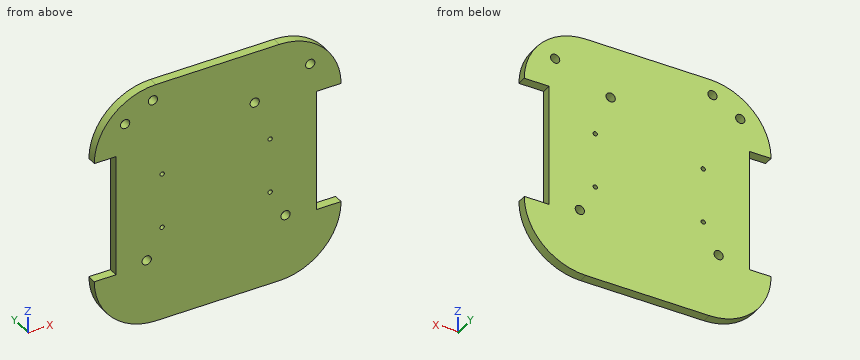
from build123d import *

# Parameters (mm, degrees)
SKETCH3_W           = 80
SKETCH3_H           = 80
BOSS_EXTRUDE1_DEPTH = 3
SKETCH4_W           = 7
SKETCH4_H           = 40
SKETCH4_W_2         = 8
CUT_EXTRUDE1_DEPTH  = 3
FILLET3_R           = 20
FILLET4_R           = 20
FILLET5_R           = 20
FILLET6_R           = 20
SKETCH6_R           = 1.5
CUT_EXTRUDE2_DEPTH  = 3
SKETCH9_R           = 1.5
CUT_EXTRUDE3_DEPTH  = 3
SKETCH10_R          = 1.5
CUT_EXTRUDE4_DEPTH  = 3
SKETCH11_R          = 0.7
CUT_EXTRUDE5_DEPTH  = 3


with BuildPart() as part:
    # Sketch3 → Boss-Extrude1 (new body)
    with BuildSketch(Plane(origin=(0, 0, 0), x_dir=(1, 0, 0), z_dir=(0, 1, 0))):
        with Locations((40, 40)):
            Rectangle(SKETCH3_W, SKETCH3_H)
    extrude(amount=BOSS_EXTRUDE1_DEPTH)

    # Sketch4 → Cut-Extrude1 (cut)
    with BuildSketch(Plane(origin=(0, 3, 0), x_dir=(1, 0, 0), z_dir=(0, 1, 0))):
        with Locations((3.5, 40)):
            Rectangle(SKETCH4_W, SKETCH4_H)
        with Locations((76, 40)):
            Rectangle(SKETCH4_W_2, SKETCH4_H)
    extrude(amount=-CUT_EXTRUDE1_DEPTH, mode=Mode.SUBTRACT)

    # Fillet3
    fillet3_edges = [part.edges().sort_by_distance(p)[0] for p in [
        (0, 1.5, -80),
    ]]
    fillet(fillet3_edges, radius=FILLET3_R - 0.0001)  # a hair under: the kernel refuses the full size

    # Fillet4
    fillet4_edges = [part.edges().sort_by_distance(p)[0] for p in [
        (80, 1.5, -80),
    ]]
    fillet(fillet4_edges, radius=FILLET4_R - 0.0001)  # a hair under: the kernel refuses the full size

    # Fillet5
    fillet5_edges = [part.edges().sort_by_distance(p)[0] for p in [
        (80, 1.5, 0),
    ]]
    fillet(fillet5_edges, radius=FILLET5_R - 0.0001)  # a hair under: the kernel refuses the full size

    # Fillet6
    fillet6_edges = [part.edges().sort_by_distance(p)[0] for p in [
        (0, 1.5, 0),
    ]]
    fillet(fillet6_edges, radius=FILLET6_R - 0.0001)  # a hair under: the kernel refuses the full size

    # Sketch6 → Cut-Extrude2 (cut)
    with BuildSketch(Plane(origin=(0, 3, 0), x_dir=(1, 0, 0), z_dir=(0, 1, 0))):
        with Locations(Location((17, 58.5, 0), (0, 0, 270))):
            Circle(SKETCH6_R)
        with Locations(Location((62, 58.5, 0), (0, 0, 270))):
            Circle(SKETCH6_R)
    extrude(amount=-CUT_EXTRUDE2_DEPTH, mode=Mode.SUBTRACT)

    # Sketch9 → Cut-Extrude3 (cut)
    with BuildSketch(Plane(origin=(0, 3, 0), x_dir=(1, 0, 0), z_dir=(0, 1, 0))):
        with Locations(Location((70, 10, 0), (0, 0, 270))):
            Circle(SKETCH9_R)
        with Locations(Location((10, 10, 0), (0, 0, 270))):
            Circle(SKETCH9_R)
    extrude(amount=-CUT_EXTRUDE3_DEPTH, mode=Mode.SUBTRACT)

    # Sketch10 → Cut-Extrude4 (cut)
    with BuildSketch(Plane(origin=(0, 3, 0), x_dir=(1, 0, 0), z_dir=(0, 1, 0))):
        with Locations(Location((19, 5, 0), (0, 0, 270))):
            Circle(SKETCH10_R)
        with Locations(Location((52, 17, 0), (0, 0, 270))):
            Circle(SKETCH10_R)
    extrude(amount=-CUT_EXTRUDE4_DEPTH, mode=Mode.SUBTRACT)

    # Sketch11 → Cut-Extrude5 (cut)
    with BuildSketch(Plane(origin=(0, 3, 0), x_dir=(1, 0, 0), z_dir=(0, 1, 0))):
        with Locations(Location((22, 49, 0), (0, 0, 270))):
            Circle(SKETCH11_R)
        with Locations(Location((22, 31, 0), (0, 0, 270))):
            Circle(SKETCH11_R)
        with Locations(Location((57, 49, 0), (0, 0, 270))):
            Circle(SKETCH11_R)
        with Locations(Location((57, 31, 0), (0, 0, 270))):
            Circle(SKETCH11_R)
    extrude(amount=-CUT_EXTRUDE5_DEPTH, mode=Mode.SUBTRACT)


solid = part.part
Design review of the part built by this model. Coordinates are the model's own, in mm. Coordinates: 2 decimals unless noted, no trailing zeros. Loops run counter-clockwise (first coordinate to the right, second up) from the corner with the lowest first, then second, coordinate; pieces in that order, holes last.
Item 1: Add section A-A (y = 1.6). Give the number of separate pieces and of enclosed holes in the cut face, and give its area (3 significant figures).
Completed:
separate pieces: 1
enclosed holes: 10
area: 5,410 mm2
Item 2: Add section B-B (x = 52). Write out the cut boundary in (y, z).
Completed:
outline: (0, -80) - (3, -80) - (3, -18.5) - (0, -18.5) - close; (0, -15.5) - (3, -15.5) - (3, 0) - (0, 0) - close
Item 3: Clearance check with flat-ended pins moving along their axes: pin 1 (4 mm diameter, centred on x = 17, z = -58.5, fed in from +Y); pin 2 (1.5 mm diameter, centred on x = 2, y = 2, fed in from -Z); pin 3 (1.5 mm diameter, centred on x = 76, y = 1, fed in from -Z); pin 4 (2.5 mm diameter, centred on x = 52, z = -17, fed in from -Y). State where each tip first meets the part, or that it passes through.
Completed:
pin 1: stops at y = 3
pin 2: stops at z = -70.12
pin 3: stops at z = -72.94
pin 4: passes through
Item 4: Wall thickness on L1, parallel to Z at x = 57, y = 0.75; L2, parallel to X at y = 0.45, z = -10.5; L3, parallel to X at y = 2.3, z = -10: over which ranges is each line inside the solid? List them lowest first.
Completed:
L1: z = -80 to -49.7, -48.3 to -31.7, -30.3 to 0
L2: x = 2.4 to 8.59, 11.41 to 68.59, 71.41 to 77.6
L3: x = 2.68 to 8.5, 11.5 to 68.5, 71.5 to 77.32
Item 5: Add section C-C (z = -17). Write out the cut boundary in (x, y).
Completed:
outline: (0.23, 0) - (50.5, 0) - (50.5, 3) - (0.23, 3) - close; (53.5, 0) - (79.77, 0) - (79.77, 3) - (53.5, 3) - close
